```python
from build123d import *

# Parameters (mm, degrees)
PAD032_DEPTH         = 10
PAD033_DEPTH         = 2.5
PAD033_DEPTH_BACK    = 4.3
FILLET011_R          = 0.5
FILLET012_R          = 1
SKETCH084_R          = 4
POCKET025_DEPTH      = 4.3010001
POCKET025_DEPTH_BACK = 4.001


with BuildPart() as part:
    # Sketch070 → Pad032 (new body, symmetric)
    with BuildSketch(Plane.YZ):
        Polygon((-12.5, 1.5), (12.5, 1.5), (15, 4), (-15, 4), align=None)
    extrude(amount=PAD032_DEPTH, both=True)

    # Sketch071 → Pad033 (join, two sides)
    with BuildSketch(Plane(origin=(0, 3, 0), x_dir=(1, 0, 0), z_dir=(0, 0, 1))) as pad033_sk:
        with BuildLine():
            ThreePointArc((7.05, 0), (0, 7.05), (-7.05, 0))
            Line((-7.05, 0), (-7.05, -7.61826472))
            ThreePointArc((-7.05, -7.61826472), (-6.0624282805, -10.3420602319), (-3.5586767903, -11.8))
            Line((-3.5586767903, -11.8), (-5.8181698251, -1.2455520409))
            ThreePointArc((5.8181698251, -1.2455520409), (0, 5.95), (-5.8181698251, -1.2455520409))
            Line((3.5586767903, -11.8), (5.8181698251, -1.2455520409))
            ThreePointArc((3.5586767903, -11.8), (6.0624283063, -10.342060201), (7.05, -7.6182646394))
            Line((7.05, 0), (7.05, -7.6182646394))
        make_face()
    extrude(amount=PAD033_DEPTH)
    extrude(pad033_sk.sketch, amount=-PAD033_DEPTH_BACK)

    # Fillet011
    fillet011_edges = [part.edges().sort_by_distance(p)[0] for p in [
        (0, 15, 4),
        (0, -15, 4),
        (-10, 0, 4),
        (10, 0, 4),
    ]]
    fillet(fillet011_edges, radius=FILLET011_R)

    # Fillet012
    fillet012_edges = [part.edges().sort_by_distance(p)[0] for p in [
        (0, 8.95, 1.5),
    ]]
    fillet(fillet012_edges, radius=FILLET012_R)

    # Sketch084 → Pocket025 (cut, two sides)
    with BuildSketch(Plane.XY) as pocket025_sk:
        Circle(SKETCH084_R)
    extrude(amount=-POCKET025_DEPTH, mode=Mode.SUBTRACT)
    extrude(pocket025_sk.sketch, amount=POCKET025_DEPTH_BACK, mode=Mode.SUBTRACT)


with BuildPart() as part_1:
    # Body023 placement: moved
    add(part.part.moved(Location((0, -2, 2.5))))


solid = part_1.part
```
Source: CAD feature listing. Evaluate the final solid. Frame: model axes, mm. A direction names the side the tool comes from. Give positions to 0.01 mm unless a question says otherwise; leave off trailing zeros. Loops run counter-clockwise (first coordinate to the right, second up) from the corner with the lowest first, then second, coordinate; pieces in that order, holes last. Notation, with made-up numbers: (40.5, 11.5) - (45.5, 11.5) arc R34 ccw to (45.5, 44.5) - close; hole circle Ø10 at (-36, -2.5). An arc over 180 degrees is marked (long way). Use CSV: the item, a comma, the result in double quotes. Start each with the question number.
1. Section A-A (x = 0). Output: boundary loops of the cut face in (y, z).
2. Reachability of faces 4 (the flat face through (-7.05, -3, 1)), 5 (the flat face through (0, -8, 4)), 6 (the cylindrical face through (3.815, -0.799, 5.232)) from +Z, -Z, +X, -X, +Y, -Y: full face, straight path, thin tool, end or side. Return the list, or none.
3. Section C-C (y = 9.75). Output: boundary loops of the cut face in (x, z).
4. Section B-B (z = 4.75). Output: boundary loops of the cut face in (x, y).
5. Section D-D (x = -7.5). Output: boundary loops of the cut face in (y, z), then the cut area to 3 significant figures.
6. Pin query (flat end, axial travel): pin 1 (1.5 mm diameter, centred on x = -4, z = 0.5, fed in from -Y); pin 2 (1.7 mm diameter, centred on y = -3, z = 1.5, fed in from +X); pin 3 (4.5 mm diameter, centred on y = -1, z = -0.5, fed in from -X). Return the tip coordinate at first contact, or that it passes through.
7. Ray query, L1, parallel to X at y = -2, z = 5.2; L2, parallel to Y at x = 0.25, z = -1; L3, parallel to X at y = -2.5, z = -0.25. Return the intervals inside material, ascending.
8. Draft query along Y for faces 1 (the cylindrical face through (0.16, 8.05, 1.14)), 2 (the flat face through (7.05, -3, 1)), 3 (the cylindrical face through (4.349, -5.67, 3.715)). Return one class per face: +Y half, -Y half, draft (parallel to the pull), parting line (faces both ways), or undercut.
Response:
1,outline,"(-16.15, 5.65) - (-14.5, 4) - (-6, 4) - (-6, 6.5) - (-15.79, 6.5) arc R0.5 ccw to start; (2, 4) - (5.95, 4) arc R1 cw to (6.95, 3) - (6.95, -1.8) - (8.05, -1.8) - (8.05, 4) - (10.5, 4) - (12.15, 5.65) arc R0.5 ccw to (11.79, 6.5) - (2, 6.5) - close"
2,face 4,"-Z, -X, +Y, -Y"
2,face 5,"-Z"
2,face 6,"+Z, -Z"
3,outline,"(-10, 4) - (10, 4) - (10, 6) arc R0.5 ccw to (9.5, 6.5) - (-9.5, 6.5) arc R0.5 ccw to (-10, 6) - close"
4,outline,"(-10, -15.25) - (10, -15.25) - (10, 11.25) - (-10, 11.25) - close; hole circle Ø8 at (0, -2)"
5,outline,"(-16.15, 5.65) - (-14.5, 4) - (10.5, 4) - (12.15, 5.65) arc R0.5 ccw to (11.79, 6.5) - (-15.79, 6.5) arc R0.5 ccw to start"
5,area,"68.1 mm²"
6,pin 1,"y = -10.8"
6,pin 2,"x = 7.05"
6,pin 3,"x = -7.05"
7,L1,"-10 to -4, 4 to 10"
7,L2,"6.94 to 8.05"
7,L3,"-7.05 to -5.34, 5.34 to 7.05"
8,face 1,"+Y half"
8,face 2,"draft"
8,face 3,"undercut"
